Geometry check sheet. Reference: the model listing, model coordinates, mm. Face numbers are marked on the shaded views. A direction names the side the tool comes from. Coordinates: 2 decimals unless noted, no trailing zeros. Loops run counter-clockwise (first coordinate to the right, second up) from the corner with the lowest first, then second, coordinate; pieces in that order, holes last. Notation, with made-up numbers: (-1, -26) - (34, -26) arc R31 cw to (34, 9) - close; hole circle Ø5 at (-23, 0). An arc over 180 degrees is marked (long way). Write item = value, one per line. Start each with the question number.
from build123d import *

# Parameters (mm, degrees)
CUT_EXTRUDE1_DEPTH        = 42.976183724
CUT_EXTRUDE1_DEPTH_BACK   = 42.976183724
SKETCH2_R                 = 3
F_6_0MM_DOWEL_HOLE1_D     = 6
F_6_0MM_DOWEL_HOLE1_DEPTH = 45
F_6_0MM_DOWEL_HOLE1_TIP   = 1.732050808
CHAMFER1_SIZE             = 1


with BuildPart() as part:
    # Sketch1 → Revolve1 (revolve)
    with BuildSketch(Plane.XY, mode=Mode.PRIVATE) as revolve1_sk:
        Polygon((-40, 0), (-40, 6), (-25, 6), (-25, 9), (25, 9), (25, 6), (40, 6), (40, 0), align=None)
    revolve(revolve1_sk.sketch.rotate(Axis((0, 0, 0), (1, 0, 0)), 90), axis=Axis((0, 0, 0), (1, 0, 0)))

    # Sketch2 → Cut-Extrude1 (cut, two sides: drawn at the far end of the back side and taken through both)
    with BuildSketch(Plane.XY.offset(-CUT_EXTRUDE1_DEPTH_BACK)):
        Circle(SKETCH2_R)
    extrude(amount=CUT_EXTRUDE1_DEPTH + CUT_EXTRUDE1_DEPTH_BACK, mode=Mode.SUBTRACT)

    # Ø6.0mm Dowel Hole1
    with Locations(Plane.ZY.offset(40)):
        with Locations((0, 0)):
            Hole(F_6_0MM_DOWEL_HOLE1_D / 2, depth=F_6_0MM_DOWEL_HOLE1_DEPTH)
            with Locations((0, 0, -(F_6_0MM_DOWEL_HOLE1_DEPTH + F_6_0MM_DOWEL_HOLE1_TIP / 2))):  # 120° drill point
                Cone(0, F_6_0MM_DOWEL_HOLE1_D / 2, F_6_0MM_DOWEL_HOLE1_TIP, mode=Mode.SUBTRACT)

    # Chamfer1
    chamfer1_edges = [part.edges().sort_by_distance(p)[0] for p in [
        (40, 0, -6),
        (-40, 0, -6),
    ]]
    chamfer(chamfer1_edges, length=CHAMFER1_SIZE)


solid = part.part
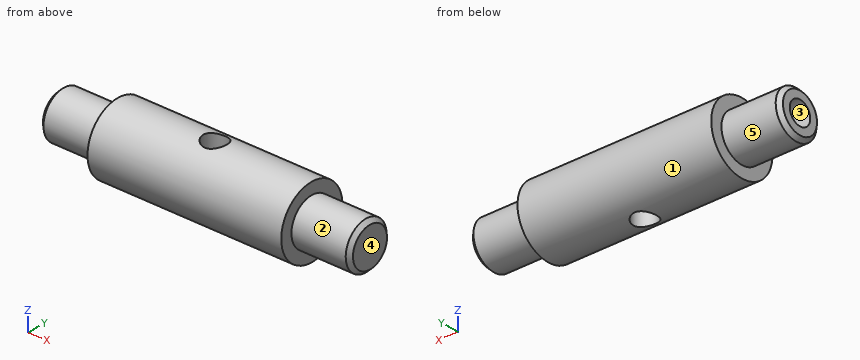
(1) Sectioned sample at C-C on z = 7. Enter the section's corners in (x, y), plus the area to 3 significant figures.
(2) Sectioned sample at A-A on x = -12. Enter the section's corners in (y, z).
(3) Sectioned sample at B-B on y = -1.25. Count the separate pieces of the cut face and the enclosed holes in it, plus the area to 3 significant figures.
(4) Draft check along Z on the marked faces 3, 4 and 5. Enter one of: pulls with the +Z half, pulls with the -Z half, needs draft (parallel to the pull), parting line crosses it, or undercut.
(5) Depth check by flat-ended pin: pin 1 (5 mm diameter, centred on x = -17.5, z = -6, fed in from -Y); pin 2 (5 mm diameter, centred on x = 26.5, y = 4, fed in from +Z); pin 3 (4 mm diameter, centred on x = -19.5, z = 5.5, fed in from +Y). Enter the tip coordinate at first touch or a pass-through.
(6) Tool access check on the marked faces 1 and 2. Record the directions out of +Z, -Z, +X, -X, +Y, -Y that give a thin tool (end or side, any length) a straight path to the whole face; none if there is none.
(7) Scan lines: line 1 (Y direction, x = -25.5, z = -0.25); line 2 (X direction, y = 0, z = -3.25); line 3 (Z direction, x = -7, y = 2.25). Record each from-to range of solid material in increasing order.
(8) Sectioned sample at D-D on x = 9.5. Enter the section's corners in (y, z), plus the area to 3 significant figures.
Working result:
q1.outline = (-25, -5.66) - (25, -5.66) - (25, 5.66) - (-25, 5.66) - close; hole circle Ø6 at (0, 0)
q1.area = 537 mm2
q2.outline = circle Ø18 at (0, 0); hole circle Ø6 at (0, 0)
q3.separate_pieces = 3
q3.enclosed_holes = 0
q3.area = 925 mm2
q4.face_3 = undercut
q4.face_4 = needs draft
q4.face_5 = parting line crosses it
q5.pin_1 = -8.29
q5.pin_2 = 8.77
q5.pin_3 = 8.29
q6.face_1 = +X, -X
q6.face_2 = +X
q7.line_1 = -5.99 to -2.99, 2.99 to 5.99
q7.line_2 = -40 to -3, 3 to 40
q7.line_3 = -8.71 to -1.98, 1.98 to 8.71
q8.outline = circle Ø18 at (0, 0)
q8.area = 254 mm2
